from build123d import *

# Parameters (mm, degrees)
F0_W          = 770
F0_H          = 505
F1_DEPTH      = 2
F1_DEPTH_BACK = 3
F2_W          = 760
F2_H          = 495
F3_DEPTH      = 61.5
F5_DEPTH      = 4
F7_DEPTH      = 25.4


with BuildPart() as f1:
    # F0 (on Top) → F1 (new body, two sides)
    with BuildSketch(Plane.XY) as f1_sk:
        Rectangle(F0_W, F0_H)
    extrude(amount=F1_DEPTH)
    extrude(f1_sk.sketch, amount=-F1_DEPTH_BACK)

    # F2 (on face) → F3 (join)
    with BuildSketch(Plane.XY.offset(2)):
        Polygon((-380, -252.5), (385, -252.5), (385, 247.5), (385, 252.5), (380, 252.5), (-385, 252.5), (-385, -247.5), (-385, -252.5), align=None)
        Rectangle(F2_W, F2_H, mode=Mode.SUBTRACT)
    extrude(amount=F3_DEPTH)

    # F4 (on face) → F5 (join)
    with BuildSketch(Plane.XY.offset(63.5)):
        Polygon((383, 250.5), (381, 250.5), (-383, 250.5), (-383, -248.5), (-383, -250.5), (-276, -250.5), (383, -250.5), (383, 248.5), align=None)
        Polygon((-381, -248.5), (-381, -247.5), (-381, 248.5), (380, 248.5), (381, 248.5), (381, 247.5), (381, -248.5), (-380, -248.5), align=None, mode=Mode.SUBTRACT)
    extrude(amount=F5_DEPTH)

    # F6 (on face) → F7 (cut)
    with BuildSketch(Plane.XZ.offset(250.5)):
        with BuildLine():
            Line((4.5, 67.5), (3.5, 67.5))
            Line((3.5, 67.5), (3.5, 66.5))
            ThreePointArc((3.5, 66.5), (4.5, 65.5), (5.5, 66.5))
            Line((5.5, 66.5), (5.5, 67.5))
            Line((5.5, 67.5), (4.5, 67.5))
        make_face()
        with BuildLine():
            Line((1.5, 67.5), (0.5, 67.5))
            Line((0.5, 67.5), (0.5, 66.5))
            ThreePointArc((0.5, 66.5), (1.5, 65.5), (2.5, 66.5))
            Line((2.5, 66.5), (2.5, 67.5))
            Line((2.5, 67.5), (1.5, 67.5))
        make_face()
        with BuildLine():
            Line((-3.5, 66.5), (-3.5, 67.5))
            Line((-3.5, 67.5), (-4.5, 67.5))
            Line((-4.5, 67.5), (-5.5, 67.5))
            Line((-5.5, 67.5), (-5.5, 66.5))
            ThreePointArc((-5.5, 66.5), (-4.5, 65.5), (-3.5, 66.5))
        make_face()
        with BuildLine():
            Line((-0.5, 66.5), (-0.5, 67.5))
            Line((-0.5, 67.5), (-1.5, 67.5))
            Line((-1.5, 67.5), (-2.5, 67.5))
            Line((-2.5, 67.5), (-2.5, 66.5))
            ThreePointArc((-2.5, 66.5), (-1.5, 65.5), (-0.5, 66.5))
        make_face()
    extrude(amount=-F7_DEPTH, mode=Mode.SUBTRACT)


solid = f1.part
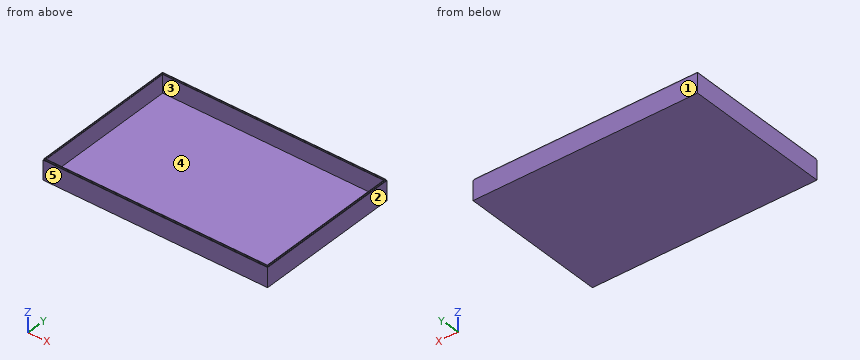
Check sheet for the modelled part. Datum: model origin and axes. Units: mm. Face numbers are marked on the shaded views. A direction names the side the tool comes from. Round coordinates to 2 decimals unless told otherwise and drop trailing zeros. Order: outer loops, then holes, each group sorted by start corner. A loop starts at its lowest first (then second) coordinate and runs counter-clockwise, first axis right, second up. Notation, with made-up numbers: M -24.5,41.25 L -15.5,41.25 A16 ccw -15.5,47.25 Z; hole C -37,24.5 d1. An arc over 180 degrees is marked long. One line per item, written item: value. Start each with the question number.
1. Section check B-B on x = 237.5. Enter the section's corners in (y, z).
2. Scan lines: line 1 along X through (y, z) = (-23, 24); line 2 along Y through (x, z) = (-23, 5.5); line 3 along X through (y, z) = (-215.5, 64.5). Record each from-to range of solid material in increasing order.
3. Gauge pin test, flat ends, axial feed: P1, Ø0.8, axis at y = -249.5, z = 67, coming from the -X side; P2, Ø3, axis at x = -147.5, z = 65.5, coming from the +Y side; P3, Ø1.1, axis at y = -250, z = 67, coming from the +X side. Record the tip position at first contact, or that the pin passes through.
4. Section check C-C on y = -193. Enter the section's corners in (x, z).
5. Section check A-A on z = 40.5. Enter the section's corners in (x, y), and give its area (4 significant figures).
6. Access from +Z, -Z, +X, -X, +Y, -Y to the whole of each face (thin tool, end or side, straight path). Record for the marked faces 4 and 5.
7. Release check for a two-part mould opening along X. For the marked faces 1, 2 and 3 record: released by +X, released by -X, zero draft, split by the parting line, or undercut.
Results found:
1. outline: M -252.5,-3 L 252.5,-3 L 252.5,63.5 L 250.5,63.5 L 250.5,67.5 L 248.5,67.5 L 248.5,63.5 L 247.5,63.5 L 247.5,2 L -247.5,2 L -247.5,63.5 L -248.5,63.5 L -248.5,67.5 L -250.5,67.5 L -250.5,63.5 L -252.5,63.5 Z
2. line 1: -385 to -380, 380 to 385
2. line 2: -252.5 to -247.5, 247.5 to 252.5
2. line 3: -383 to -381, 381 to 383
3. P1: x = -383
3. P2: y = 250.5
3. P3: x = 383
4. outline: M -385,-3 L 385,-3 L 385,63.5 L 383,63.5 L 383,67.5 L 381,67.5 L 381,63.5 L 380,63.5 L 380,2 L -380,2 L -380,63.5 L -381,63.5 L -381,67.5 L -383,67.5 L -383,63.5 L -385,63.5 Z
5. outline: M -385,-252.5 L 385,-252.5 L 385,252.5 L -385,252.5 Z; hole M -380,-247.5 L 380,-247.5 L 380,247.5 L -380,247.5 Z
5. area: 12,650 mm^2
6. face 4: +Z
6. face 5: +Z, -Z, +X, -X, -Y
7. face 1: zero draft
7. face 2: released by +X
7. face 3: undercut
